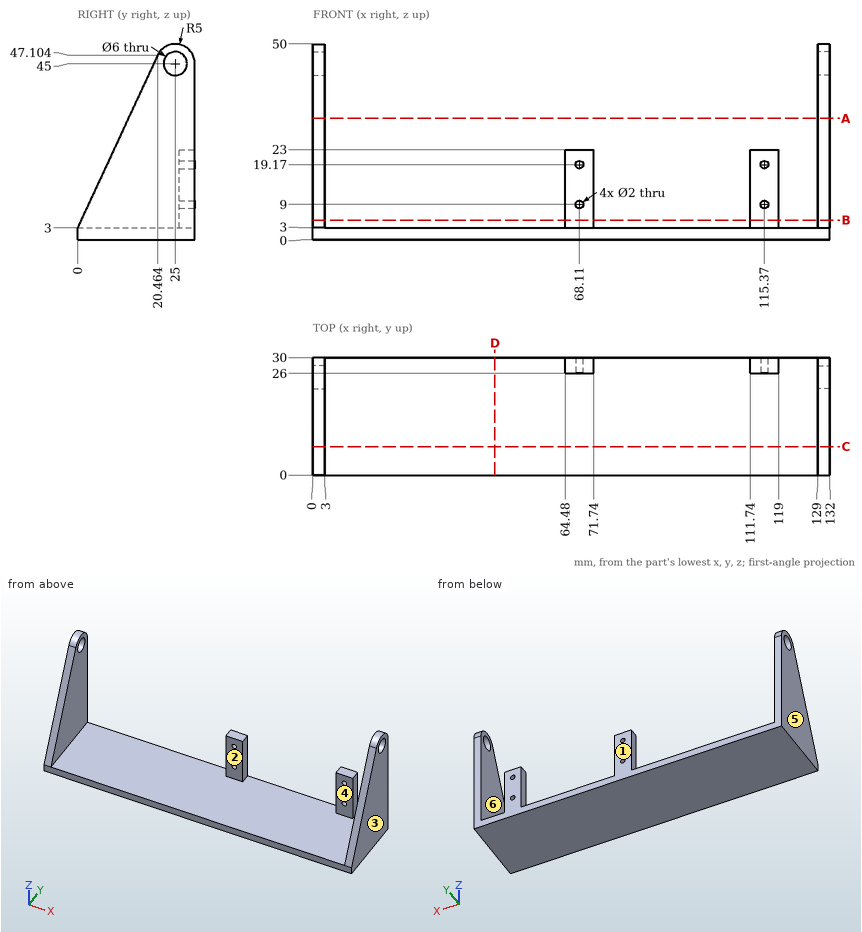
Part print with two shaded views. Sizes in mm from the minimum x, y, z corner. A direction names the side the tool comes from. Round coordinates to 2 decimals unless told otherwise and drop trailing zeros. Loops run counter-clockwise (first coordinate to the right, second up) from the corner with the lowest first, then second, coordinate; pieces in that order, holes last. Notation, with made-up numbers: (89, 10.25) - (116, 10.25) arc R24 cw to (116, 21.25) - close; hole circle Ø9 at (82, -38.75). An arc over 180 degrees is marked (long way). Put each result on its own line as item: value.
1. Slice it at A-A on z = 31. List the corners of the cut face in (x, y), and give its area (3 significant figures).
Geometry check:
outline: (0, 12.99) - (3, 12.99) - (3, 30) - (0, 30) - close; (129, 12.99) - (132, 12.99) - (132, 30) - (129, 30) - close
area: 102 mm²
2. Pin check, flat tips, straight feed: P1, Ø2.5, axis at x = 115.37, z = 19.17, coming from the -Y side; P2, Ø1.2, axis at x = 69, y = 27.5, coming from the +Z side. Stop position of each tip, or through.
Geometry check:
P1: y = 26
P2: z = 23
3. Wall check: line 1 (X direction, y = 22.5, z = 17); line 2 (Z direction, x = 115.37, y = 28.3); line 3 (Z direction, x = 1.75, y = 25). Give the ranges that are in metal, low to high.
Geometry check:
line 1: 0 to 3, 129 to 132
line 2: 0 to 8, 10 to 18.17, 20.17 to 23
line 3: 0 to 42, 48 to 50
4. Two-plate mould, pull along X, no slides. Class the marked faces 1, 2 and 3: released by +X, released by -X, zero draft, split by the parting line, or undercut.
Geometry check:
face 1: zero draft
face 2: undercut
face 3: released by +X
5. Slice it at D-D on x = 46.5. List the corners of the cut face in (y, z).
Geometry check:
outline: (0, 0) - (30, 0) - (30, 3) - (0, 3) - close
6. Slice it at B-B on z = 5. List the corners of the cut face in (x, y).
Geometry check:
outline: (0, 0.93) - (3, 0.93) - (3, 30) - (0, 30) - close; (64.48, 26) - (71.74, 26) - (71.74, 30) - (64.48, 30) - close; (111.74, 26) - (119, 26) - (119, 30) - (111.74, 30) - close; (129, 0.93) - (132, 0.93) - (132, 30) - (129, 30) - close
7. 3-axis set-ups, long thin cutter, end or side, ignore diameter. For the marked faces 4, 5 and 6: which of +Z, -Z, +X, -X, +Y, -Y reach the whole face in a straight line?
Geometry check:
face 4: +Z, -Y
face 5: +Z, -Z, -X, +Y, -Y
face 6: +Z, +Y, -Y
8. Slice it at C-C on y = 7.25. List the corners of the cut face in (x, z) (1 decimal).
Geometry check:
outline: (0, 0) - (132, 0) - (132, 18.6) - (129, 18.6) - (129, 3) - (3, 3) - (3, 18.6) - (0, 18.6) - close
